The model under review builds one solid part; all positions refer to its coordinate system, in mm. Coordinates: 2 decimals unless noted, no trailing zeros. Order: outer loops, then holes, each group sorted by start corner. A loop starts at its lowest first (then second) coordinate and runs counter-clockwise, first axis right, second up. Notation, with made-up numbers: (46, 71.5) -> (85, 71.5) arc R13 cw to (85, 80.5) -> close; hole circle Ø10 at (-10.75, 14). An arc over 180 degrees is marked (long way). Answer as CSV lines item,"result". Start each with the question number.
from build123d import *

# Parameters (mm, degrees)
F0_R     = 15
F1_DEPTH = 25.4
F2_DEPTH = 600
F3_DEPTH = 25.4
F4_DEPTH = 25.4
F5_DEPTH = 25.4


with BuildPart() as f1:
    # F0 (on Top) → F1 (new body)
    with BuildSketch(Plane.XY):
        Circle(F0_R)
    extrude(amount=F1_DEPTH)

    # F2 (add): a face of the model
    f2_faces = [f1.faces().sort_by_distance(p)[0] for p in [
        (0, 0, 25.4),
    ]]
    extrude(f2_faces, amount=F2_DEPTH)

    # F3 (add): a face of the model
    f3_faces = [f1.faces().sort_by_distance(p)[0] for p in [
        (0, 0, 625.4),
    ]]
    extrude(f3_faces, amount=F3_DEPTH)

    # F4 (add): faces of the model
    f4_faces = [f1.faces().sort_by_distance(p)[0] for p in [
        (0, 0, 650.8),
        (0, 0, 0),
    ]]
    extrude(f4_faces, amount=F4_DEPTH, dir=(0, 0, 1))

    # F5 (add): a face of the model
    f5_faces = [f1.faces().sort_by_distance(p)[0] for p in [
        (0, 0, 676.2),
    ]]
    extrude(f5_faces, amount=F5_DEPTH)


solid = f1.part
1) Consider section B-B (y = -7.25). Give the boundary of the cut face in (x, z), plus the area to 3 significant figures.
2) Insertion check: pin 1 Ø10 at (y, z) = (8.5, 477.5) entering from -X; pin 2 Ø3 at (x, z) = (-4.5, 599.5) entering from -Y; pin 3 Ø3 at (x, z) = (6, 234) entering from -Y. Each pin has a flat end and moves straight along its axis. Give the tip position at first contact, or say it passes through.
3) Consider section A-A (z = 173). Give the boundary of the cut face in (x, y), plus the area to 3 significant figures.
4) Wall thickness on L1, parallel to X at y = -0.5, z = 496.5; L2, parallel to X at y = -2.5, z = 392; L3, parallel to Y at x = -12.5, z = 161: over which ranges is each line inside the solid? List them lowest first. Write a range as [from, to].
5) Consider section C-C (x = 8.5). Give the boundary of the cut face in (y, z), plus the area to 3 significant figures.
Result:
1,outline,"(-13.13, 0) -> (13.13, 0) -> (13.13, 701.6) -> (-13.13, 701.6) -> close"
1,area,"18,400 mm2"
2,pin 1,"x = -14.59"
2,pin 2,"y = -14.7"
2,pin 3,"y = -14.31"
3,outline,"circle Ø30 at (0, 0)"
3,area,"707 mm2"
4,L1,"[-14.99, 14.99]"
4,L2,"[-14.79, 14.79]"
4,L3,"[-8.29, 8.29]"
5,outline,"(-12.36, 0) -> (12.36, 0) -> (12.36, 701.6) -> (-12.36, 701.6) -> close"
5,area,"17,300 mm2"
